```python
from build123d import *

# Parameters (mm, degrees)
F0_R     = 2.15265
F0_R_2   = 1.7272
F0_R_3   = 9.525
F0_R_4   = 3.96875
F0_R_5   = 7.9375
F1_DEPTH = 5.08


with BuildPart() as f1:
    # F0 (on Top) → F1 (new body)
    with BuildSketch(Plane.XY):
        with BuildLine():
            Line((0, 23.8125), (-193.597083, 23.8125))
            Line((-193.597083, 23.8125), (-203.122083, 23.8125))
            Line((-203.122083, 23.8125), (-203.122083, -101.6))
            Line((-203.122083, -101.6), (23.8125, -101.6))
            Line((23.8125, -101.6), (23.8125, -90.805))
            Line((23.8125, -90.805), (23.8125, 0))
            ThreePointArc((23.8125, 0), (16.83798, 16.83798), (0, 23.8125))
        make_face()
        with Locations((-188.834583, -96.2025)):
            Circle(F0_R, mode=Mode.SUBTRACT)
        with Locations((-198.359583, -40.653914)):
            Circle(F0_R, mode=Mode.SUBTRACT)
        with Locations((9.525, -96.2025)):
            Circle(F0_R, mode=Mode.SUBTRACT)
        with Locations((-198.359583, 19.05)):
            Circle(F0_R, mode=Mode.SUBTRACT)
        with Locations((-81.238881, -31.663497)):
            Circle(F0_R_2, mode=Mode.SUBTRACT)
        with Locations((-60.568717, -26.406832)):
            Circle(F0_R_2, mode=Mode.SUBTRACT)
        with Locations((-73.532132, -18.700083)):
            Circle(F0_R_3, mode=Mode.SUBTRACT)
        with Locations((-86.495546, -10.993334)):
            Circle(F0_R_2, mode=Mode.SUBTRACT)
        with Locations((-12.909118, -12.909118)):
            Circle(F0_R_4, mode=Mode.SUBTRACT)
        with Locations((12.909118, -12.909118)):
            Circle(F0_R_2, mode=Mode.SUBTRACT)
        with Locations((-65.825382, -5.736669)):
            Circle(F0_R_2, mode=Mode.SUBTRACT)
        Circle(F0_R_5, mode=Mode.SUBTRACT)
        with Locations((-12.909118, 12.909118)):
            Circle(F0_R_2, mode=Mode.SUBTRACT)
        with Locations((12.909118, 12.909118)):
            Circle(F0_R_4, mode=Mode.SUBTRACT)
    extrude(amount=F1_DEPTH)


solid = f1.part
```
Geometry check sheet. Reference: the model listing, model coordinates, mm. Coordinates: 2 decimals unless noted, no trailing zeros. Order: outer loops, then holes, each group sorted by start corner. A loop starts at its lowest first (then second) coordinate and runs counter-clockwise, first axis right, second up. Notation, with made-up numbers: (-38, 80) - (-26, 80) arc R30 ccw to (-26, 114) - close; hole circle Ø6 at (47.25, -2.75). An arc over 180 degrees is marked (long way). Answer as a JSON object with one key per item and string values. Group by question number.
Item 1: Draft check along Y on faces 1 (the face through (-100, 23.812, 3)), 2 (the face through (-91, -101.6, 3)), 3 (the face through (-9.243, -14.429, 2.504)), 4 (the face through (-91, -38, 5.08)). Enter one of: +Y half, -Y half, draft (parallel to the pull), parting line (faces both ways), or undercut.
Item 2: Scan lines: probe 1 along X at (y, z) = (13.5, 1.65); probe 2 along X at (y, z) = (-31.5, 2.1); probe 3 along Y at (x, z) = (0, 1.35). Record each from-to range of solid material in increasing order.
Item 3: Sectioned sample at B-B, the plane z = 1.1. Give the number of separate pieces and of enclosed holes in the cut face, and give its area (3 significant figures).
Item 4: Sectioned sample at A-A, the plane y = 19.05. Record the cut outline in (x, z), and give its area (3 significant figures).
Resolved:
{
 "1": {"face 1": "+Y half", "face 2": "-Y half", "face 3": "undercut", "face 4": "draft"},
 "2": {"probe 1": "-203.12 to -14.53, -11.29 to 8.98, 16.83 to 19.62", "probe 2": "-203.12 to -82.96, -79.52 to 23.81", "probe 3": "-101.6 to -7.94, 7.94 to 23.81"},
 "3": {"separate pieces": "1", "enclosed holes": "14", "area": "27,600 mm^2"},
 "4": {"outline": "(-203.12, 0) - (-200.51, 0) - (-200.51, 5.08) - (-203.12, 5.08) - close; (-196.21, 0) - (14.29, 0) - (14.29, 5.08) - (-196.21, 5.08) - close", "area": "1,080 mm^2"}
}
